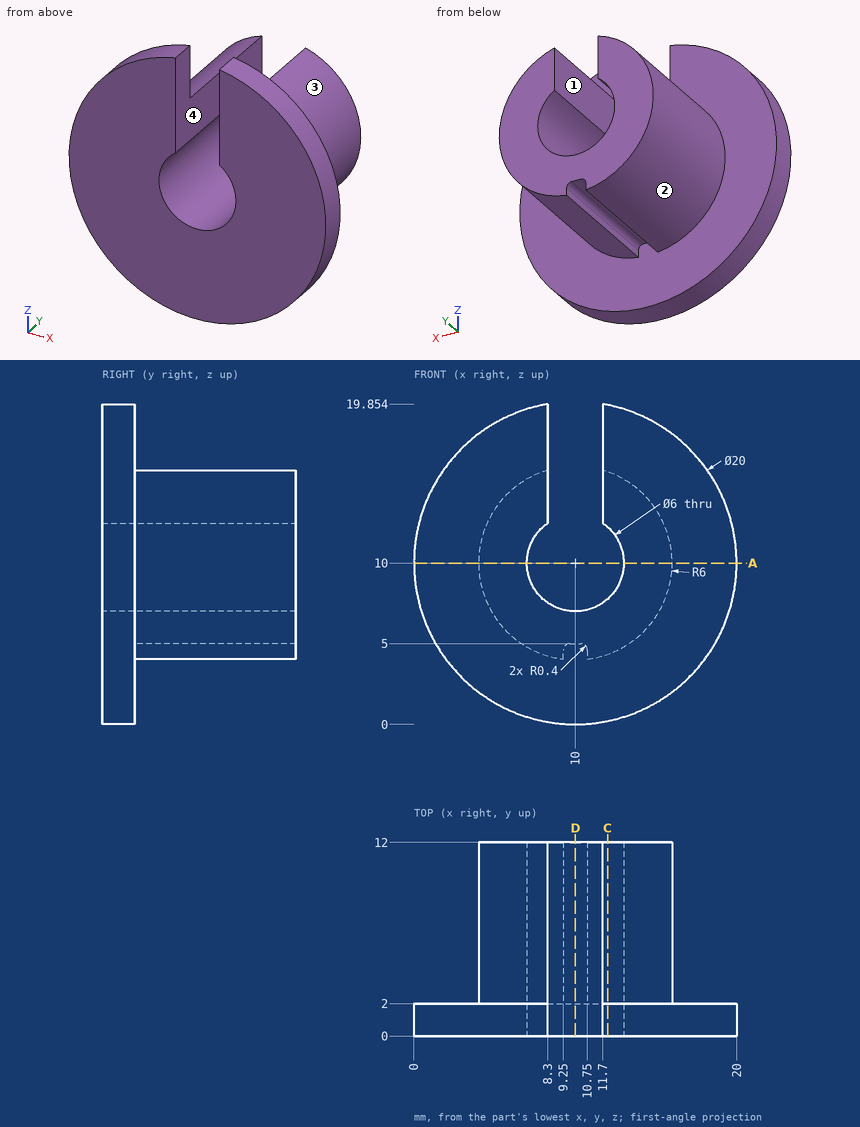
The drawing under review shows one solid part. Ordinate dimensions are in mm from its lowest x, y, z. Coordinates: 2 decimals unless noted, no trailing zeros. Loops run counter-clockwise (first coordinate to the right, second up) from the corner with the lowest first, then second, coordinate; pieces in that order, holes last.
Item 1: Add section A-A (z = 10). Write out the cut boundary in (x, y).
Completed:
outline: (0, 0) - (7, 0) - (7, 12) - (4, 12) - (4, 2) - (0, 2) - close; (13, 0) - (20, 0) - (20, 2) - (16, 2) - (16, 12) - (13, 12) - close
Item 2: Add section D-D (x = 10). Write out the cut boundary in (y, z), and give its area (3 significant figures).
Completed:
outline: (0, 0) - (2, 0) - (2, 5) - (12, 5) - (12, 7) - (0, 7) - close
area: 34.0 mm2
Item 3: Wall thickness on L1, parallel to X at y = 6, z = 10; L2, parallel to Y at x = 15.75, z = 4.75; L3, parallel to X at y = 3.75, z = 11.25: over which ranges is each line inside the solid? List them lowest first.
Completed:
L1: x = 4 to 7, 13 to 16
L2: y = 0 to 2
L3: x = 4.13 to 7.27, 12.73 to 15.87
Item 4: Clearance check with flat-ended pins moving along their axes: pin 1 (5 mm diameter, centred on y = 7.5, z = 4, fed in from +X); pin 2 (4 mm diameter, centred on x = 15.5, y = 7.5, fed in from +Z); pin 3 (1 mm diameter, centred on y = 1.5, z = 14, fed in from +X). State where each tip first meets the part, or that it passes through.
Completed:
pin 1: stops at x = 14.87
pin 2: stops at z = 14.87
pin 3: stops at x = 19.37
Item 5: Add section C-C (x = 12). Write out the cut boundary in (y, z).
Completed:
outline: (0, 0.2) - (2, 0.2) - (2, 4.34) - (12, 4.34) - (12, 7.76) - (0, 7.76) - close; (0, 12.24) - (12, 12.24) - (12, 15.66) - (2, 15.66) - (2, 19.8) - (0, 19.8) - close
Item 6: Draft analysis for pull direction X (two halves, no side actions). For the marked faces 1, 2, 3 and 4, state which applies: pulls with the +X half, pulls with the -X half, needs draft (parallel to the pull), parting line crosses it, or undercut.
Completed:
face 1: undercut
face 2: pulls with the -X half
face 3: pulls with the +X half
face 4: undercut
